from build123d import *

# Parameters (mm, degrees)
BOSS_EXTRUDE1_DEPTH            = 2.521826736
SKETCH2_R                      = 11.136118556
BOSS_EXTRUDE2_DEPTH            = 50.8
SKETCH3_W                      = 86.137031446
SKETCH3_H                      = 59.748072355
BOSS_EXTRUDE3_DEPTH            = 50.8
CUT_EXTRUDE1_DEPTH             = 109.100560925
CUT_EXTRUDE2_REACH             = 110.101
SKETCH6_R                      = 3.175
CUT_EXTRUDE3_DEPTH             = 118.741599385
CUT_EXTRUDE3_DEPTH_BACK        = 118.741599385
SKETCH8_W                      = 38.1
SKETCH8_H                      = 12.7
CUT_EXTRUDE4_REACH             = 119.073
SKETCH9_W                      = 12.477031446
SKETCH9_H                      = 38.1
CUT_EXTRUDE4_DIRECTION_2_DEPTH = 118.073406314
SKETCH10_W                     = 12.477031446
SKETCH10_H                     = 15.24
CUT_EXTRUDE5_DEPTH             = 109.100560925


with BuildPart() as part:
    # Sketch1 → Boss-Extrude1 (new body)
    with BuildSketch(Plane.XY):
        with BuildLine():
            Line((-11.136118556, 0), (-11.136118556, 25.4))
            Line((-11.136118556, 25.4), (11.136118556, 25.4))
            Line((11.136118556, 25.4), (11.136118556, 0))
            ThreePointArc((11.136118556, 0), (0, 11.136118556), (-11.136118556, 0))
        make_face()
    boss_extrude1 = extrude(amount=BOSS_EXTRUDE1_DEPTH)

    # Sketch2 → Boss-Extrude2 (add)
    with BuildSketch(Plane.XY):
        Circle(SKETCH2_R)
    extrude(amount=BOSS_EXTRUDE2_DEPTH)

    # Sketch3 → Boss-Extrude3 (add)
    with BuildSketch(Plane.XY):
        with Locations((0, 55.274036178)):
            Rectangle(SKETCH3_W, SKETCH3_H)
    extrude(amount=BOSS_EXTRUDE3_DEPTH)

    # Sketch4 → Cut-Extrude1 (cut, through all)
    with BuildSketch(Plane.XY.offset(50.8)):
        Polygon((20.431484277, 85.148072355), (20.431484277, 59.748072355), (31.75, 59.748072355), (31.75, 34.29), (-31.75, 34.29), (-31.75, 59.748072355), (-20.431484277, 59.748072355), (-20.431484277, 85.148072355), align=None)
    extrude(amount=-CUT_EXTRUDE1_DEPTH, mode=Mode.SUBTRACT)

    # Mirror1: Boss-Extrude1 across plane
    add(boss_extrude1.mirror(Plane(origin=(0, 0, 12.7), x_dir=(1, 0, 0), z_dir=(0, 0, -1))))

    # Sketch6 → Cut-Extrude2 (cut, up to next)
    with BuildSketch(Plane.XY.offset(50.8), mode=Mode.PRIVATE) as cut_extrude2_sk1:
        Circle(SKETCH6_R)
    cut_extrude2_tool1 = extrude(cut_extrude2_sk1.sketch, amount=-CUT_EXTRUDE2_REACH, mode=Mode.PRIVATE) & part.part
    add(cut_extrude2_tool1.solids().sort_by_distance((0, 0, 50.8))[0], mode=Mode.SUBTRACT)

    # Sketch8 → Cut-Extrude3 (cut, two sides: drawn at the far end of the back side and taken through both)
    with BuildSketch(Plane(origin=(-20.431484277, 0, 0), x_dir=(0, 0, -1), z_dir=(1, 0, 0)).offset(-CUT_EXTRUDE3_DEPTH_BACK)):
        with Locations((-25.4, 72.448072355)):
            Rectangle(SKETCH8_W, SKETCH8_H)
    extrude(amount=CUT_EXTRUDE3_DEPTH + CUT_EXTRUDE3_DEPTH_BACK, mode=Mode.SUBTRACT)

    # Sketch9 → Cut-Extrude4 (cut, up to next)
    with BuildSketch(Plane(origin=(0, 85.148072355, 0), x_dir=(1, 0, 0), z_dir=(0, 1, 0)), mode=Mode.PRIVATE) as cut_extrude4_sk1:
        with Locations((-31.75, -25.4)):
            Rectangle(SKETCH9_W, SKETCH9_H)
    cut_extrude4_tool1 = extrude(cut_extrude4_sk1.sketch, amount=-CUT_EXTRUDE4_REACH, mode=Mode.PRIVATE) & part.part
    # Sketch9 → Cut-Extrude4 (cut, up to next)
    with BuildSketch(Plane(origin=(0, 85.148072355, 0), x_dir=(1, 0, 0), z_dir=(0, 1, 0)), mode=Mode.PRIVATE) as cut_extrude4_sk2:
        with Locations((31.75, -25.4)):
            Rectangle(SKETCH9_W, SKETCH9_H)
    cut_extrude4_tool2 = extrude(cut_extrude4_sk2.sketch, amount=-CUT_EXTRUDE4_REACH, mode=Mode.PRIVATE) & part.part
    add(cut_extrude4_tool1.solids().sort_by_distance((-31.75, 85.148072, 25.4))[0], mode=Mode.SUBTRACT)
    add(cut_extrude4_tool2.solids().sort_by_distance((31.75, 85.148072, 25.4))[0], mode=Mode.SUBTRACT)

    # Sketch9 → Cut-Extrude4 direction 2 (cut)
    with BuildSketch(Plane(origin=(0, 85.148072355, 0), x_dir=(1, 0, 0), z_dir=(0, 1, 0))):
        with Locations((-31.75, -25.4)):
            Rectangle(SKETCH9_W, SKETCH9_H)
        with Locations((31.75, -25.4)):
            Rectangle(SKETCH9_W, SKETCH9_H)
    extrude(amount=CUT_EXTRUDE4_DIRECTION_2_DEPTH, mode=Mode.SUBTRACT)

    # Sketch10 → Cut-Extrude5 (cut, through all)
    with BuildSketch(Plane.XY.offset(50.8)):
        with Locations((-31.75, 72.448072355)):
            Rectangle(SKETCH10_W, SKETCH10_H)
        with Locations((31.75, 72.448072355)):
            Rectangle(SKETCH10_W, SKETCH10_H)
    extrude(amount=-CUT_EXTRUDE5_DEPTH, mode=Mode.SUBTRACT)


solid = part.part
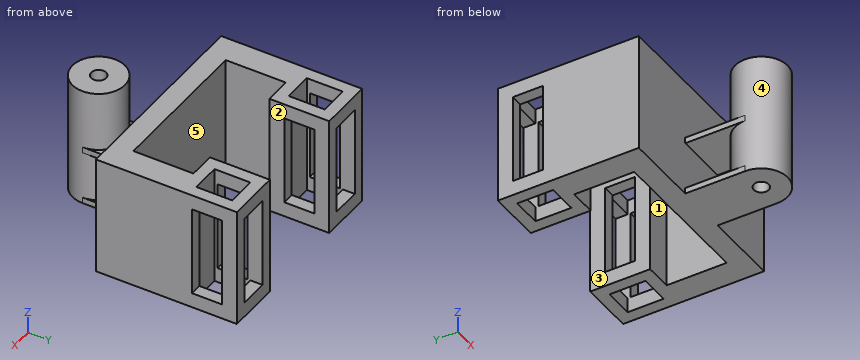
Here's how the part is built. I have some questions about the finished solid (model axes, mm). Face numbers are marked on the shaded views. A direction names the side the tool comes from. Round coordinates to 2 decimals unless told otherwise and drop trailing zeros. Write each loop counter-clockwise with the first axis right and the second up, starting at its lowest first coordinate (ties: lowest second). Pieces come first, ordered by that corner, then holes.
1. If we mould it in two halves opening along Y, with no side actions, what happens to the marked faces 1 and 2? For each: released by +Y, released by -Y, zero draft, split by the parting line, or undercut.
2. Suppose I cut it at B-B (y = 24). List the corners of the cut face in (x, z) for me.
3. Suppose I cut it at A-A (x = 0). List the corners of the cut face in (y, z) for me (3 decimals), and give its area (3 significant figures).
4. For the marked faces 3, 4 and 5, which set-ups out of +Z, -Z, +X, -X, +Y, -Y let a thin tool reach every point of the face, with its end or its side?
5. Will these pins go through, and if not, where does the flat tip stop? pin 1 Ø10 at (x, y) = (-6, 0.5) entering from -Z; pin 2 Ø1.9 at (x, z) = (30, 4) entering from -Y; pin 3 Ø2 at (y, z) = (2, 13.5) entering from +X; pin 4 Ø6 at (x, z) = (-29.5, 33) entering from +Y.
6. Suppose I cut it at C-C (x = 29). List the corners of the cut face in (y, z) for me, and give its area (3 significant figures).
7. Suppose I cut it at D-D (z = 29). State how many separate pieces and enclosed holes the cut face has, and give its area (3 significant figures).
8. I need wall thicknesses on L1, parallel to Y at x = 25, z = 23; L2, parallel to Y at x = 0, z = 27 (3 decimals); L3, parallel to Z at x = 10.5, y = 21. Which ranges of each line are inside material? Lowest first, please.
Answer sheet:
1. face 1: undercut
1. face 2: zero draft
2. outline: (-11.14, 0) - (11.14, 0) - (11.14, 2.52) - (-11.14, 2.52) - close; (-11.14, 22.88) - (11.14, 22.88) - (11.14, 25.4) - (-11.14, 25.4) - close
3. outline: (-11.136, 0) - (-3.175, 0) - (-3.175, 50.8) - (-11.136, 50.8) - close; (3.175, 0) - (34.29, 0) - (34.29, 50.8) - (25.4, 50.8) - (25.4, 25.4) - (11.136, 25.4) - (11.136, 50.8) - (3.175, 50.8) - close; hole (11.136, 2.522) - (25.4, 2.522) - (25.4, 22.878) - (11.136, 22.878) - close
3. area: 1,330 mm2
4. face 3: +Z, -Z, +Y
4. face 4: none
4. face 5: +Z, -Z
5. pin 1: stops at z = 0
5. pin 2: stops at y = 25.4
5. pin 3: stops at x = 11.09
5. pin 4: stops at y = 64.83
6. outline: (25.4, 0) - (34.29, 0) - (34.29, 50.8) - (25.4, 50.8) - close; (59.75, 0) - (64.83, 0) - (64.83, 50.8) - (59.75, 50.8) - close; (80.07, 0) - (85.15, 0) - (85.15, 6.35) - (80.07, 6.35) - close; (80.07, 44.45) - (85.15, 44.45) - (85.15, 50.8) - (80.07, 50.8) - close
6. area: 774 mm2
7. separate pieces: 6
7. enclosed holes: 1
7. area: 2,080 mm2
8. L1: y = 25.4 to 34.29, 59.75 to 66.1, 78.8 to 85.15
8. L2: y = -11.136 to -3.175, 3.175 to 11.136, 25.4 to 34.29
8. L3: z = 0 to 2.52, 22.88 to 25.4
